Here's how the part is built. I have some questions about the finished solid (model axes, mm). A direction names the side the tool comes from. Round coordinates to 2 decimals unless told otherwise and drop trailing zeros. Order: outer loops, then holes, each group sorted by start corner. A loop starts at its lowest first (then second) coordinate and runs counter-clockwise, first axis right, second up. Notation, with made-up numbers: (24.5, 36.5) -> (35.5, 36.5) arc R9 cw to (35.5, 48.5) -> close; hole circle Ø4 at (78.25, 86). An arc over 180 degrees is marked (long way). One line per item, written item: value.
```python
from build123d import *

# Parameters (mm, degrees)
F1_DEPTH = 150
F2_T     = -5
F4_DEPTH = 25


with BuildPart() as f1:
    # F0 (on Front) → F1 (new body)
    with BuildSketch(Plane.XZ):
        Polygon((-12.2474321396, 63.0875647986), (-59.0572801928, 17.9894703241), (-43.4061087422, -45.0980944746), (19.0549107617, -63.0875647986), (65.8647588149, -17.9894703241), (50.2135873642, 45.0980944746), align=None)
    extrude(amount=F1_DEPTH)

    # F2
    f2_openings = [f1.faces().sort_by_distance(p)[0] for p in [
        (3.403739, -150, 0),
    ]]
    offset(amount=F2_T, openings=f2_openings)

    # F3 (on face) → F4 (cut)
    with BuildSketch(Plane(origin=(-15.3186231144, 0, -53.1876036307), x_dir=(0.9609387616, 0, -0.2767610819), z_dir=(-0.2767610819, 0, -0.9609387616))):
        Polygon((-5.047660324, 59.1908805072), (11.5892304007, 59.1908805072), (21.9621621023, 72.1981254462), (18.26010564, 88.4178945857), (3.2707850383, 95.6363709407), (-11.7185355634, 88.4178945857), (-15.4205920256, 72.1981254462), align=None)
    extrude(amount=-F4_DEPTH, mode=Mode.SUBTRACT)


solid = f1.part
```
Q1. I need wall thicknesses on line 1 along Y through (x, z) = (15, 10); line 2 along Z through (x, y) = (13.5, -101); line 3 along Z through (x, y) = (4, -8). Which ranges of each line are inside material? Lowest first, please.
Answers:
line 1: -5 to 0
line 2: -61.49 to -56.28, 50.47 to 55.67
line 3: -58.75 to -53.55, 53.2 to 58.41
Q2. I want a section at D-D on y = -69. Write out the boundary of the cut face in (x, z), then the cut area to 3 significant figures.
Answers:
outline: (-59.06, 17.99) -> (-43.41, -45.1) -> (-27.69, -49.63) -> (-26.3, -44.82) -> (-39.25, -41.09) -> (-53.51, 16.39) -> (-10.86, 57.48) -> (46.06, 41.09) -> (60.32, -16.39) -> (17.66, -57.48) -> (4.72, -53.76) -> (3.33, -58.56) -> (19.05, -63.09) -> (65.86, -17.99) -> (50.21, 45.1) -> (-12.25, 63.09) -> close
area: 1,700 mm2
Q3. For P1, Ø1, axis at x = -45, z = -8.5, coming from the +Y side; P2, Ø1.5, axis at x = -26, z = 6, coming from the -Y side; P3, Ø12, axis at y = -118, z = 15.5, coming from the -X side; P4, Ø2, axis at y = -36.5, z = 0.5, coming from the +X side, each with a flat end and sliding along its axis, tell me the tip position at first contact or that it passes through.
Answers:
P1: y = 0
P2: y = -5
P3: x = -59.06
P4: x = 61.53
Q4. I want a section at B-B on z = 50.5. Write out the boundary of the cut face in (x, y).
Answers:
outline: (-25.31, -150) -> (-18.11, -150) -> (-18.11, -5) -> (13.39, -5) -> (13.39, -150) -> (31.46, -150) -> (31.46, 0) -> (-25.31, 0) -> close
Q5. I want a section at A-A on y = -40. Write out the boundary of the cut face in (x, z), then the cut area to 3 significant figures.
Answers:
outline: (-59.06, 17.99) -> (-43.41, -45.1) -> (19.05, -63.09) -> (65.86, -17.99) -> (50.21, 45.1) -> (-12.25, 63.09) -> close; hole (-53.51, 16.39) -> (-39.25, -41.09) -> (17.66, -57.48) -> (60.32, -16.39) -> (46.06, 41.09) -> (-10.86, 57.48) -> close
area: 1,860 mm2
Q6. Which directions (+Z, -Z, +X, -X, +Y, -Y) give clear straight access to the entire face, cutting with the end or side of a thin tool? Please do faces 5 (the face through (38.69, -76.48, -37.23)), 6 (the face through (-24.541, -65.786, -47.966)), 7 (the face through (-4.191, -91.977, -53.827)).
Answers:
face 5: -Y
face 6: -Z
face 7: none
Q7. I want a section at C-C on x = 30.5. Write out the boundary of the cut face in (y, z), then the cut area to 3 significant figures.
Answers:
outline: (-150, -52.06) -> (0, -52.06) -> (0, 50.78) -> (-150, 50.78) -> (-150, 45.57) -> (-5, 45.57) -> (-5, -45.12) -> (-150, -45.12) -> close
area: 2,280 mm2
Q8. If we mould it in two halves opening along X, with no side actions, what happens to faces 1 (the face through (40, -150, -37)), 2 (the face through (42.132, -73.95, -40.854)), 3 (the face through (-27.65, -80.42, -47.07)), 4 (the face through (-12, -59.191, -52))? For each: pulls with the +X half, pulls with the -X half, needs draft (parallel to the pull), parting line crosses it, or undercut.
Answers:
face 1: needs draft
face 2: pulls with the +X half
face 3: undercut
face 4: undercut
